Geometry check sheet. Reference: drawing and pictorial views, mm from the part's lowest x, y, z. A direction names the side the tool comes from. Give positions to 0.01 mm unless a question says otherwise; leave off trailing zeros. Write each loop counter-clockwise with the first axis right and the second up, starting at its lowest first coordinate (ties: lowest second). Pieces come first, ordered by that corner, then holes. Notation, with made-up numbers: (5.5, 7) -> (25.5, 7) arc R23 ccw to (25.5, 42) -> close; hole circle Ø7 at (87, 65.25). An arc over 180 degrees is marked (long way). Use a Markdown table: item, result. Add a question column.
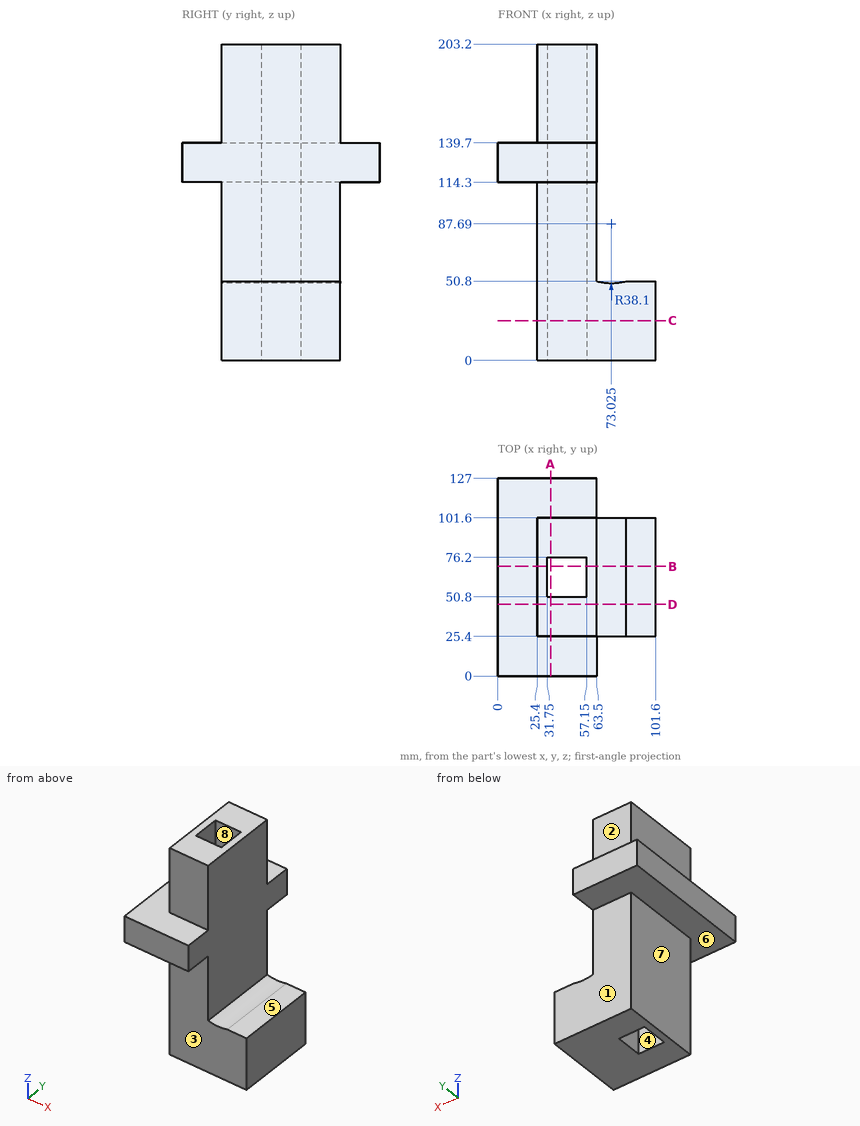
1) Sectioned sample at D-D, the plane y = 46. Enter the section's corners in (x, z) (3 decimals), and give its area (3 significant figures).
2) Sectioned sample at A-A, the plane x = 34. Enter the section's corners in (y, z).
3) Sectioned sample at C-C, the plane z = 25.5. Enter the section's corners in (x, y).
4) Gauge pin test, flat ends, axial feed: P1, Ø1, axis at y = 27, z = 143.5, coming from the +X side; P2, Ø15, axis at x = 95, y = 50.5, coming from the +Z side; P3, Ø12, axis at y = 25.5, z = 44.5, coming from the -X side. Record the tip position at first contact, or that the pin passes through.
5) Material ranges on probe 1 along X at (y, z) = (67.5, 14); probe 2 along X at (y, z) = (68, 77.5); probe 3 along Z at (x, y) = (53.5, 117.5), recorded low to high. Write a range as [from, to].
6) Tool access check on the marked faces 1, 2, 3, 4 and 5. Record the directions out of +Z, -Z, +X, -X, +Y, -Y that give a thin tool (end or side, any length) a straight path to the whole face; none if there is none.
7) Draft check along X on the marked faces 6, 7 and 8. Enter one of: +X half, -X half, draft (parallel to the pull), parting line (faces both ways), or undercut.
8) Sectioned sample at B-B, the plane y = 70.5. Enter the section's corners in (x, z) (3 decimals), and give its area (3 significant figures).
Check values:
| question | item | result |
|---|---|---|
| 1 | outline | (0, 114.3) -> (25.4, 114.3) -> (25.4, 0) -> (101.6, 0) -> (101.6, 50.8) -> (82.55, 50.8) arc R38.1 cw to (63.5, 50.8) -> (63.5, 203.2) -> (25.4, 203.2) -> (25.4, 139.7) -> (0, 139.7) -> close |
| 1 | area | 10,300 mm² |
| 2 | outline | (0, 114.3) -> (25.4, 114.3) -> (25.4, 0) -> (50.8, 0) -> (50.8, 203.2) -> (25.4, 203.2) -> (25.4, 139.7) -> (0, 139.7) -> close; (76.2, 0) -> (101.6, 0) -> (101.6, 114.3) -> (127, 114.3) -> (127, 139.7) -> (101.6, 139.7) -> (101.6, 203.2) -> (76.2, 203.2) -> close |
| 3 | outline | (25.4, 25.4) -> (101.6, 25.4) -> (101.6, 101.6) -> (25.4, 101.6) -> close; hole (31.75, 50.8) -> (57.15, 50.8) -> (57.15, 76.2) -> (31.75, 76.2) -> close |
| 4 | P1 | x = 63.5 |
| 4 | P2 | z = 50.8 |
| 4 | P3 | x = 25.4 |
| 5 | probe 1 | [25.4, 31.75], [57.15, 101.6] |
| 5 | probe 2 | [25.4, 31.75], [57.15, 63.5] |
| 5 | probe 3 | [114.3, 139.7] |
| 6 | face 1 | -Z, +X, -X, +Y |
| 6 | face 2 | +Z, +X, -X, +Y |
| 6 | face 3 | -Z, +X, -X, -Y |
| 6 | face 4 | +Z, -Z |
| 6 | face 5 | +Z, +X, +Y, -Y |
| 7 | face 6 | draft |
| 7 | face 7 | -X half |
| 7 | face 8 | undercut |
| 8 | outline | (0, 114.3) -> (25.4, 114.3) -> (25.4, 0) -> (31.75, 0) -> (31.75, 203.2) -> (25.4, 203.2) -> (25.4, 139.7) -> (0, 139.7) -> close; (57.15, 0) -> (101.6, 0) -> (101.6, 50.8) -> (82.55, 50.8) arc R38.1 cw to (63.5, 50.8) -> (63.5, 203.2) -> (57.15, 203.2) -> close |
| 8 | area | 5,150 mm² |
